```python
from build123d import *

# Parameters (mm, degrees)
F1_DEPTH = 75
F2_W     = 10
F2_H     = 12.5
F3_DEPTH = 11


with BuildPart() as f1:
    # F0 (on Front) → F1 (new body, symmetric)
    with BuildSketch(Plane.XZ):
        with BuildLine():
            Line((100, 13.75), (100, 16.25))
            Line((100, 16.25), (-100, 16.25))
            Line((-100, 16.25), (-100, -16.25))
            Line((-100, -16.25), (70, -16.25))
            ThreePointArc((70, -16.25), (91.2132034356, -7.4632034356), (100, 13.75))
        make_face()
    extrude(amount=F1_DEPTH, both=True)

    # F2 (on face) → F3 (cut)
    with BuildSketch(Plane.XY.offset(16.25)):
        Polygon((87.5, -62.5), (87.5, 62.5), (-87.5, 62.5), (-87.5, 36.7867040902), (-41, 36.7867040902), (-33.5, 36.7867040902), (-33.5, 28.7867040902), (-38.5, 28.7867040902), (-38.5, 31.7867040902), (-46, 31.7867040902), (-87.5, 31.7867040902), (-87.5, 4.8), (-92.5, 1.8), (-100, 1.8), (-100, -1.8), (-92.5, -1.8), (-87.5, -4.8), (-87.5, -31.2132959098), (-38.5, -31.2132959098), (-38.5, -28.2132959098), (-33.5, -28.2132959098), (-33.5, -36.2132959098), (-41, -36.2132959098), (-46, -36.2132959098), (-87.5, -36.2132959098), (-87.5, -62.5), (-77.5, -62.5), align=None)
        with BuildLine():
            Line((-77.3618234992, 52.5), (-74.3618234992, 52.5))
            Line((-74.3618234992, 52.5), (60.6381765008, 52.5))
            Line((60.6381765008, 52.5), (74.5, 52.5))
            Line((74.5, 52.5), (77.5, 52.5))
            Line((77.5, 52.5), (77.5, 49.5))
            Line((77.5, 49.5), (77.5, -52.5))
            Line((77.5, -52.5), (60.6381765008, -52.5))
            Line((60.6381765008, -52.5), (-77.5, -52.5))
            Line((-77.5, -52.5), (-77.5, -49.5))
            Line((-77.5, -49.5), (60.6381765008, -49.5))
            Line((60.6381765008, -49.5), (69.5, -49.5))
            ThreePointArc((69.5, -49.5), (73.0355339059, -48.0355339059), (74.5, -44.5))
            Line((74.5, -44.5), (74.5, 44.5))
            ThreePointArc((74.5, 44.5), (73.0355339059, 48.0355339059), (69.5, 49.5))
            Line((69.5, 49.5), (60.6381765008, 49.5))
            Line((60.6381765008, 49.5), (57.6381765008, 49.5))
            Line((57.6381765008, 49.5), (-74.3618234992, 49.5))
            Line((-74.3618234992, 49.5), (-77.3618234992, 49.5))
            Line((-77.3618234992, 49.5), (-77.3618234992, 52.5))
        make_face(mode=Mode.SUBTRACT)
        Polygon((40, -25), (40, 0), (40, 25), (40, 37.5), (50, 37.5), (50, 25), (50, -25), (50, -37.5), (40, -37.5), align=None, mode=Mode.SUBTRACT)
        with Locations((45, 31.25)):
            Rectangle(F2_W, F2_H)
        with Locations((45, -31.25)):
            Rectangle(F2_W, F2_H)
        Polygon((40, 25), (40, 0), (40, -25), (50, -25), (50, 25), align=None)
        with BuildLine():
            Line((60.6381765008, 52.5), (-74.3618234992, 52.5))
            Line((-74.3618234992, 52.5), (-77.3618234992, 52.5))
            Line((-77.3618234992, 52.5), (-77.3618234992, 49.5))
            Line((-77.3618234992, 49.5), (-74.3618234992, 49.5))
            Line((-74.3618234992, 49.5), (57.6381765008, 49.5))
            Line((57.6381765008, 49.5), (60.6381765008, 49.5))
            Line((60.6381765008, 49.5), (69.5, 49.5))
            ThreePointArc((69.5, 49.5), (73.0355339059, 48.0355339059), (74.5, 44.5))
            Line((74.5, 44.5), (74.5, -44.5))
            ThreePointArc((74.5, -44.5), (73.0355339059, -48.0355339059), (69.5, -49.5))
            Line((69.5, -49.5), (60.6381765008, -49.5))
            Line((60.6381765008, -49.5), (-77.5, -49.5))
            Line((-77.5, -49.5), (-77.5, -52.5))
            Line((-77.5, -52.5), (60.6381765008, -52.5))
            Line((60.6381765008, -52.5), (77.5, -52.5))
            Line((77.5, -52.5), (77.5, 49.5))
            Line((77.5, 49.5), (77.5, 52.5))
            Line((77.5, 52.5), (74.5, 52.5))
            Line((74.5, 52.5), (60.6381765008, 52.5))
        make_face()
    extrude(amount=-F3_DEPTH, mode=Mode.SUBTRACT)


solid = f1.part
```
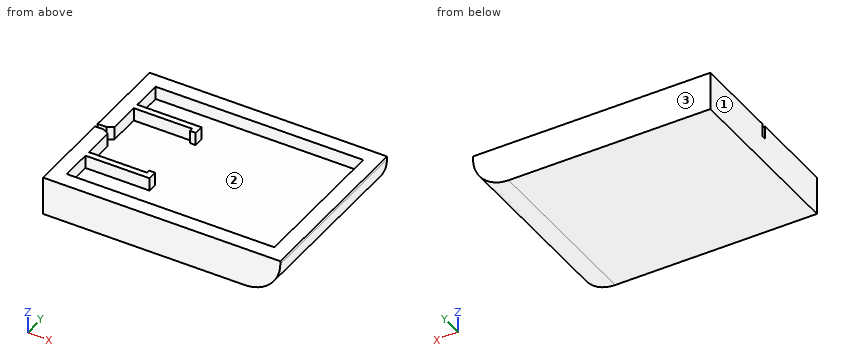
Here's how the part is built. I have some questions about the finished solid (model axes, mm). Face numbers are marked on the shaded views. Round coordinates to 2 decimals unless told otherwise and drop trailing zeros. Order: outer loops, then holes, each group sorted by start corner. A loop starts at its lowest first (then second) coordinate and runs counter-clockwise, first axis right, second up. Notation, with made-up numbers: M -18,0 L 4,0 A9 ccw 4,7 Z; hole C -16,19.5 d6. An arc over 180 degrees is marked long. Answer in a Markdown table with one row per item.
Item 1: Imagine slicing it at B-B, the plane x = 20.5. Write out the boundary of the cut face in (y, z), and give its area (3 significant figures).
A:
| item | result |
|---|---|
| outline | M -75,-16.25 L 75,-16.25 L 75,16.25 L 62.5,16.25 L 62.5,5.25 L -62.5,5.25 L -62.5,16.25 L -75,16.25 Z |
| area | 3,500 mm2 |
Item 2: If I drill on L1, parallel to Y at x = -50, z = 8; L2, parallel to Z at x = -31, y = 11.5; L3, parallel to Y at x = -23, z = 6.5, over which ranges is the centre line in solid material (lowest first)? Write a range as from..to.
A:
| item | result |
|---|---|
| L1 | y = -75..-62.5, -36.21..-31.21, 31.79..36.79, 62.5..75 |
| L2 | z = -16.25..5.25 |
| L3 | y = -75..-62.5, 62.5..75 |
Item 3: Thinking about a two-plate mould opening in X: for the marked faces 1, 2 and 3, which applies, +X half, -X half, draft (parallel to the pull), parting line (faces both ways), or undercut?
A:
| item | result |
|---|---|
| face 1 | -X half |
| face 2 | undercut |
| face 3 | draft |
Item 4: Imagine slicing it at C-C, the plane z = 10.5. Write out the boundary of the cut face in (x, y), and give its area (3 significant figures).
A:
| item | result |
|---|---|
| outline | M -100,-75 L 99.82,-75 L 99.82,75 L -100,75 L -100,1.8 L -92.5,1.8 L -87.5,4.8 L -87.5,31.79 L -38.5,31.79 L -38.5,28.79 L -33.5,28.79 L -33.5,36.79 L -87.5,36.79 L -87.5,62.5 L 87.5,62.5 L 87.5,-62.5 L -87.5,-62.5 L -87.5,-36.21 L -33.5,-36.21 L -33.5,-28.21 L -38.5,-28.21 L -38.5,-31.21 L -87.5,-31.21 L -87.5,-4.8 L -92.5,-1.8 L -100,-1.8 Z |
| area | 8,610 mm2 |
Item 5: I'm going to push flat-ended pins straight in: pin 1 (5.5 mm diameter, centred on y = 19, z = 11.5, fed in from +X); pin 2 (8 mm diameter, centred on x = -10.5, y = -52.5, fed in from +Z). Where does each tip first touch, or does it pass through?
A:
| item | result |
|---|---|
| pin 1 | stops at x = 100 |
| pin 2 | stops at z = 5.25 |
Item 6: Imagine slicing it at D-D, the plane x = -49. Write out the boundary of the cut face in (y, z).
A:
| item | result |
|---|---|
| outline | M -75,-16.25 L 75,-16.25 L 75,16.25 L 62.5,16.25 L 62.5,5.25 L 36.79,5.25 L 36.79,16.25 L 31.79,16.25 L 31.79,5.25 L -31.21,5.25 L -31.21,16.25 L -36.21,16.25 L -36.21,5.25 L -62.5,5.25 L -62.5,16.25 L -75,16.25 Z |
Item 7: Imagine slicing it at A-A, the plane y = 53.5. Write out the boundary of the cut face in (x, z).
A:
| item | result |
|---|---|
| outline | M -100,-16.25 L 70,-16.25 A30 ccw 100,13.75 L 100,16.25 L 87.5,16.25 L 87.5,5.25 L -87.5,5.25 L -87.5,16.25 L -100,16.25 Z |
